from build123d import *

# Parameters (mm, degrees)
F0_R     = 14.2875
F1_DEPTH = 3.175


with BuildPart() as f1:
    # F0 (on Top) → F1 (new body)
    with BuildSketch(Plane.XY):
        with BuildLine():
            Line((-101.720522, 36.347288), (-103.024984, 36.578738))
            ThreePointArc((-103.024984, 36.578738), (-104.9987, 36.105304), (-105.995444, 34.337198))
            Line((-105.995444, 34.337198), (-106.130744, 33.019289))
            ThreePointArc((-106.130744, 33.019289), (-106.875934, 31.46823), (-108.438793, 30.748117))
            Line((-108.438793, 30.748117), (-109.758711, 30.634062))
            ThreePointArc((-109.758711, 30.634062), (-111.542641, 29.665924), (-112.047802, 27.700088))
            Line((-112.047802, 27.700088), (-111.837391, 26.392068))
            ThreePointArc((-111.837391, 26.392068), (-112.155746, 24.700991), (-113.478973, 23.600917))
            Line((-113.478973, 23.600917), (-114.724396, 23.149128))
            ThreePointArc((-114.724396, 23.149128), (-116.196967, 21.752264), (-116.17612, 19.722667))
            Line((-116.17612, 19.722667), (-115.634338, 18.513674))
            ThreePointArc((-115.634338, 18.513674), (-115.504162, 16.797823), (-116.497582, 15.392757))
            Line((-116.497582, 15.392757), (-117.583636, 14.634023))
            ThreePointArc((-117.583636, 14.634023), (-118.644496, 12.903626), (-118.09906, 10.948582))
            Line((-118.09906, 10.948582), (-117.262829, 9.921009))
            ThreePointArc((-117.262829, 9.921009), (-116.692994, 8.297315), (-117.288906, 6.68301))
            Line((-117.288906, 6.68301), (-118.141578, 5.669038))
            ThreePointArc((-118.141578, 5.669038), (-118.718431, 3.723032), (-117.685578, 1.975774))
            Line((-117.685578, 1.975774), (-116.611885, 1.199647))
            ThreePointArc((-116.611885, 1.199647), (-115.641224, -0.221237), (-115.799017, -1.934769))
            Line((-115.799017, -1.934769), (-116.360201, -3.134879))
            ThreePointArc((-116.360201, -3.134879), (-116.413734, -5.163876), (-114.963851, -6.584277))
            Line((-114.963851, -6.584277), (-113.725866, -7.056066))
            ThreePointArc((-113.725866, -7.056066), (-112.420528, -8.177308), (-112.12945, -9.873293))
            Line((-112.12945, -9.873293), (-112.360901, -11.177755))
            ThreePointArc((-112.360901, -11.177755), (-111.887466, -13.151472), (-110.11936, -14.148215))
            Line((-110.11936, -14.148215), (-108.801451, -14.283515))
            ThreePointArc((-108.801451, -14.283515), (-107.250392, -15.028705), (-106.53028, -16.591565))
            Line((-106.53028, -16.591565), (-106.416224, -17.911482))
            ThreePointArc((-106.416224, -17.911482), (-105.448086, -19.695412), (-103.48225, -20.200573))
            Line((-103.48225, -20.200573), (-102.17423, -19.990162))
            ThreePointArc((-102.17423, -19.990162), (-100.483153, -20.308517), (-99.383079, -21.631745))
            Line((-99.383079, -21.631745), (-98.93129, -22.877167))
            ThreePointArc((-98.93129, -22.877167), (-97.534426, -24.349739), (-95.504829, -24.328891))
            Line((-95.504829, -24.328891), (-94.295837, -23.787109))
            ThreePointArc((-94.295837, -23.787109), (-92.579985, -23.656934), (-91.174919, -24.650353))
            Line((-91.174919, -24.650353), (-90.416186, -25.736407))
            ThreePointArc((-90.416186, -25.736407), (-88.685789, -26.797267), (-86.730744, -26.251831))
            Line((-86.730744, -26.251831), (-85.703171, -25.4156))
            ThreePointArc((-85.703171, -25.4156), (-84.079478, -24.845765), (-82.465172, -25.441677))
            Line((-82.465172, -25.441677), (-81.4512, -26.29435))
            ThreePointArc((-81.4512, -26.29435), (-79.505194, -26.871202), (-77.757936, -25.838349))
            Line((-77.757936, -25.838349), (-76.981809, -24.764656))
            ThreePointArc((-76.981809, -24.764656), (-75.560925, -23.793995), (-73.847393, -23.951788))
            Line((-73.847393, -23.951788), (-72.647283, -24.512972))
            ThreePointArc((-72.647283, -24.512972), (-70.618286, -24.566505), (-69.197886, -23.116622))
            Line((-69.197886, -23.116622), (-68.726097, -21.878637))
            ThreePointArc((-68.726097, -21.878637), (-67.604854, -20.573299), (-65.908869, -20.282221))
            Line((-65.908869, -20.282221), (-64.604407, -20.513672))
            ThreePointArc((-64.604407, -20.513672), (-62.630691, -20.040237), (-61.633947, -18.272131))
            Line((-61.633947, -18.272131), (-61.498647, -16.954222))
            ThreePointArc((-61.498647, -16.954222), (-60.753457, -15.403164), (-59.190598, -14.683051))
            Line((-59.190598, -14.683051), (-57.87068, -14.568995))
            ThreePointArc((-57.87068, -14.568995), (-56.08675, -13.600857), (-55.581589, -11.635021))
            Line((-55.581589, -11.635021), (-55.792, -10.327001))
            ThreePointArc((-55.792, -10.327001), (-55.473645, -8.635924), (-54.150418, -7.53585))
            Line((-54.150418, -7.53585), (-52.904995, -7.084061))
            ThreePointArc((-52.904995, -7.084061), (-51.432424, -5.687197), (-51.453271, -3.6576))
            Line((-51.453271, -3.6576), (-51.995053, -2.448608))
            ThreePointArc((-51.995053, -2.448608), (-52.125228, -0.732756), (-51.131809, 0.672309))
            Line((-51.131809, 0.672309), (-50.045755, 1.431043))
            ThreePointArc((-50.045755, 1.431043), (-48.984895, 3.16144), (-49.530331, 5.116484))
            Line((-49.530331, 5.116484), (-50.366562, 6.144058))
            ThreePointArc((-50.366562, 6.144058), (-50.936397, 7.767751), (-50.340485, 9.382056))
            Line((-50.340485, 9.382056), (-49.487813, 10.396028))
            ThreePointArc((-49.487813, 10.396028), (-48.91096, 12.342034), (-49.943813, 14.089293))
            Line((-49.943813, 14.089293), (-51.017506, 14.86542))
            ThreePointArc((-51.017506, 14.86542), (-51.988167, 16.286303), (-51.830374, 17.999836))
            Line((-51.830374, 17.999836), (-51.26919, 19.199945))
            ThreePointArc((-51.26919, 19.199945), (-51.215657, 21.228943), (-52.66554, 22.649343))
            Line((-52.66554, 22.649343), (-53.903525, 23.121132))
            ThreePointArc((-53.903525, 23.121132), (-55.208863, 24.242375), (-55.499941, 25.93836))
            Line((-55.499941, 25.93836), (-55.26849, 27.242822))
            ThreePointArc((-55.26849, 27.242822), (-55.741925, 29.216538), (-57.510031, 30.213282))
            Line((-57.510031, 30.213282), (-58.82794, 30.348581))
            ThreePointArc((-58.82794, 30.348581), (-60.378998, 31.093772), (-61.099111, 32.656631))
            Line((-61.099111, 32.656631), (-61.213167, 33.976548))
            ThreePointArc((-61.213167, 33.976548), (-62.181305, 35.760479), (-64.147141, 36.26564))
            Line((-64.147141, 36.26564), (-65.455161, 36.055229))
            ThreePointArc((-65.455161, 36.055229), (-67.146238, 36.373584), (-68.246312, 37.696811))
            Line((-68.246312, 37.696811), (-68.698101, 38.942234))
            ThreePointArc((-68.698101, 38.942234), (-70.094965, 40.414805), (-72.124562, 40.393958))
            Line((-72.124562, 40.393958), (-73.333554, 39.852176))
            ThreePointArc((-73.333554, 39.852176), (-75.049406, 39.722), (-76.454472, 40.71542))
            Line((-76.454472, 40.71542), (-77.213205, 41.801474))
            ThreePointArc((-77.213205, 41.801474), (-78.943602, 42.862333), (-80.898647, 42.316898))
            Line((-80.898647, 42.316898), (-81.92622, 41.480667))
            ThreePointArc((-81.92622, 41.480667), (-83.549913, 40.910832), (-85.164219, 41.506743))
            Line((-85.164219, 41.506743), (-86.178191, 42.359416))
            ThreePointArc((-86.178191, 42.359416), (-88.124197, 42.936268), (-89.871455, 41.903416))
            Line((-89.871455, 41.903416), (-90.647582, 40.829723))
            ThreePointArc((-90.647582, 40.829723), (-92.068465, 39.859062), (-93.781998, 40.016855))
            Line((-93.781998, 40.016855), (-94.982107, 40.578039))
            ThreePointArc((-94.982107, 40.578039), (-97.011105, 40.631572), (-98.431505, 39.181689))
            Line((-98.431505, 39.181689), (-98.903294, 37.943704))
            ThreePointArc((-98.903294, 37.943704), (-100.024537, 36.638366), (-101.720522, 36.347288))
        make_face()
        with Locations((-83.814695, 8.032533)):
            Circle(F0_R, mode=Mode.SUBTRACT)
    extrude(amount=F1_DEPTH)


solid = f1.part
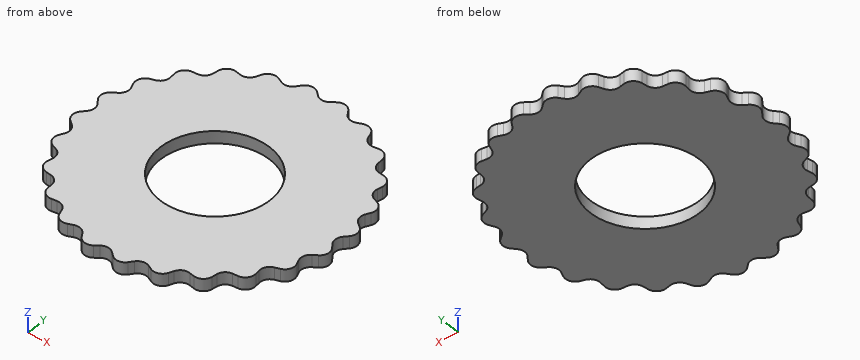
The listing builds one solid part. Answer for the finished solid, in the listing's coordinates (mm). Give positions to 0.01 mm unless a question says otherwise; leave off trailing zeros. Order: outer loops, then holes, each group sorted by start corner. A loop starts at its lowest first (then second) coordinate and runs counter-clockwise, first axis right, second up. Notation, with made-up numbers: (3.5, -19.75) - (55.5, -19.75) arc R21 ccw to (55.5, 18.25) - close; hole circle Ø10 at (54.25, 52.5). An arc over 180 degrees is marked (long way). One line per item, written item: value. Start each with the question number.
1) Find the intervals of material crossed by L1, parallel to Y at x = -73, z = 2.2; L2, parallel to X at y = 11.5, z = 1.65; L3, parallel to Y at x = -79, z = 2.6, in increasing order.
2) A cutting plane is placed at B-B on y = -4.5. Give the vertices of the cut face in (x, z) (3 decimals), then the cut area to 3 significant figures.
3) Given pin 1 Ø2 at (x, y) = (-109.5, -15.5) entering from -Z; pin 2 Ø1 at (x, z) = (-66.5, 1) entering from -Y, each flat-ended and moving along its own axis, determine where each tip first touches the part or whether it passes through.
4) A cutting plane is placed at A-A on x = -75. Give the vertices of the cut face in (y, z) (3 decimals), then the cut area to 3 significant figures.
5) A cutting plane is placed at D-D on y = -15.5. Give the vertices of the cut face in (x, z) (3 decimals), then the cut area to 3 significant figures.
6) A cutting plane is placed at C-C on x = -104.5. Give the vertices of the cut face in (y, z) (3 decimals).
Answer sheet:
1. L1: y = -24.35 to -1.3, 17.37 to 40
1. L2: x = -118.44 to -97.68, -69.95 to -48.95
1. L3: y = -26.76 to -5.42, 21.48 to 42.87
2. outline: (-116.583, 0) - (-90.675, 0) - (-90.675, 3.175) - (-116.583, 3.175) - close; (-76.954, 0) - (-51.239, 0) - (-51.239, 3.175) - (-76.954, 3.175) - close
2. area: 164 mm2
3. pin 1: passes through
3. pin 2: stops at y = -20.33
4. outline: (-23.714, 0) - (-3.212, 0) - (-3.212, 3.175) - (-23.714, 3.175) - close; (19.277, 0) - (39.709, 0) - (39.709, 3.175) - (19.277, 3.175) - close
4. area: 130 mm2
5. outline: (-106.885, 0) - (-60.847, 0) - (-60.847, 3.175) - (-106.885, 3.175) - close
5. area: 146 mm2
6. outline: (-20.157, 0) - (36.399, 0) - (36.399, 3.175) - (-20.157, 3.175) - close
